Design review of the part built by this model. Coordinates are the model's own, in mm. Give positions to 0.01 mm unless a question says otherwise; leave off trailing zeros. Order: outer loops, then holes, each group sorted by start corner. A loop starts at its lowest first (then second) coordinate and runs counter-clockwise, first axis right, second up.
```python
from build123d import *

# Parameters (mm, degrees)
BOSS_EXTRUDE2_DEPTH      = 10
SKETCH2_R                = 7.5
CUT_EXTRUDE2_DEPTH       = 10
ELBOW_MOTOR_HOLDER_DEPTH = 5


with BuildPart() as part:
    # Sketch1 → Boss-Extrude2 (new body)
    with BuildSketch(Plane.XY):
        with BuildLine():
            Line((20, 160), (-20, 160))
            Line((-20, 160), (-20, -140.000000151))
            ThreePointArc((-20, -140.000000151), (7.5e-08, -160), (20, -140))
            Line((20, -140), (20, 160))
        make_face()
    extrude(amount=BOSS_EXTRUDE2_DEPTH)

    # Sketch2 → Cut-Extrude2 (cut)
    with BuildSketch(Plane(origin=(0, 0, 0), x_dir=(-1, 0, 0), z_dir=(0, 0, -1))):
        with Locations((0, 150)):
            Circle(SKETCH2_R)
    extrude(amount=-CUT_EXTRUDE2_DEPTH, mode=Mode.SUBTRACT)

    # Sketch3 → elbow motor holder (add, symmetric)
    with BuildSketch(Plane(origin=(0, 0, 0), x_dir=(0, 0, -1), z_dir=(1, 0, 0))):
        with BuildLine():
            Line((-33.808782217, 113.808782217), (-33.808782217, 103.808782217))
            ThreePointArc((-33.808782217, 103.808782217), (-10, 80), (-33.808782217, 56.191217783))
            Line((-33.808782217, 56.191217783), (-33.808782217, 46.191217783))
            ThreePointArc((-33.808782217, 46.191217783), (0, 80), (-33.808782217, 113.808782217))
        make_face()
    extrude(amount=ELBOW_MOTOR_HOLDER_DEPTH, both=True)


solid = part.part
```
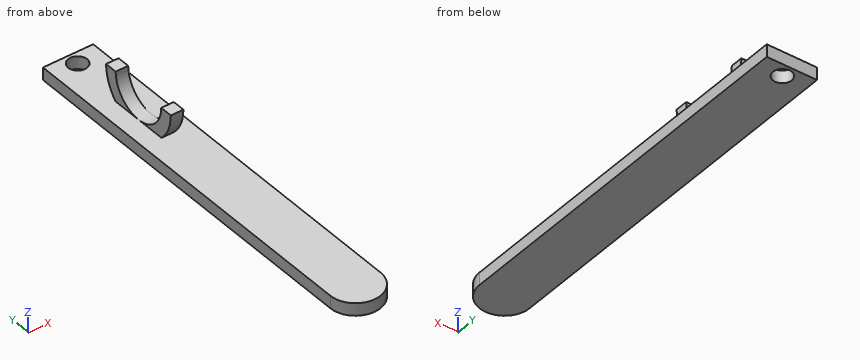
1. For line 1 along Z through (x, y) = (16.5, -43.5); line 2 along Y through (x, z) = (1, 17.5); line 3 along Y through (x, z) = (0, 3), list the stretches that pass through material, from the lowest coordinate up.
Recorded:
line 1: z = 0 to 10
line 2: y = 50.38 to 62.65, 97.35 to 109.62
line 3: y = -160 to 142.5, 157.5 to 160
2. Take a section at D-D (z = 7). State the section outline as (x, y) points, then the cut area to 3 significant figures.
Recorded:
outline: (-20, -140) arc R20 ccw to (20, -140) - (20, 160) - (-20, 160) - close; hole circle Ø15 at (0, 150)
area: 12,500 mm2
3. Take a section at C-C (z = 26). State the section outline as (x, y) points, then the cut area to 3 significant figures.
Recorded:
outline: (-5, 47.11) - (5, 47.11) - (5, 57.51) - (-5, 57.51) - close; (-5, 102.49) - (5, 102.49) - (5, 112.89) - (-5, 112.89) - close
area: 208 mm2
4. Take a section at B-B (y = 150). State the section outline as (x, z) points, then the cut area to 3 significant figures.
Recorded:
outline: (-20, 0) - (-7.5, 0) - (-7.5, 10) - (-20, 10) - close; (7.5, 0) - (20, 0) - (20, 10) - (7.5, 10) - close
area: 250 mm2
5. For pin 1 (19 mm diameter, centred on y = 56, z = 20.5, fed in from -X); pin 2 (1 mm diameter, centred on x = -2, z = 27.5, fed in from +Y); pin 3 (2 mm diameter, centred on x = 16, y = -2.5, fed in from +Z); pin 4 (5 mm diameter, centred on y = -48.5, z = 14.5, fed in from +X), all flat-tipped, find the tip position at first contact; note any pin that passes through.
Recorded:
pin 1: stops at x = -5
pin 2: stops at y = 113.31
pin 3: stops at z = 10
pin 4: passes through
6. Take a section at A-A (x = 0). State the section outline as (y, z) points, then the cut area to 3 significant figures.
Recorded:
outline: (-160, 0) - (142.5, 0) - (142.5, 10) - (104, 10) arc R33.81 ccw to (113.81, 33.81) - (103.81, 33.81) arc R23.81 cw to (56.19, 33.81) - (46.19, 33.81) arc R33.81 ccw to (56, 10) - (-160, 10) - close; (157.5, 0) - (160, 0) - (160, 10) - (157.5, 10) - close
area: 3,620 mm2
